For this review, use the dimensioned drawing (mm, ordinates from the lowest corner) and the shaded views. Coordinates: 2 decimals unless noted, no trailing zeros. Loops run counter-clockwise (first coordinate to the right, second up) from the corner with the lowest first, then second, coordinate; pieces in that order, holes last. Notation, with made-up numbers: (10.25, -27) - (50.25, -27) arc R15 ccw to (50.25, -7) - close; hole circle Ø8 at (-7, 46.5). An arc over 180 degrees is marked (long way). One line per item, written item: value. Start each with the question number.
1. We need section C-C, the plane y = 3.9. Give the boundary of the cut face in (x, z).
2. We need section A-A, the plane x = 8.8. Give the boundary of the cut face in (y, z), then the cut area to 3 significant figures.
3. We need section B-B, the plane z = 33.1. Give the boundary of the cut face in (x, y).
4. To check wall thickness, follow line 1 (X direction, y = 0.45, z = 33.1); line 2 (Z direction, x = 8.8, y = 1.35); line 3 (Y direction, x = 1.75, z = 44). State the ranges of each line that lie inside material, in increasing order.
5. Insertion check: P1, Ø1, axis at y = 0.5, z = 12.5, coming from the -X side; P2, Ø10, axis at x = 9, z = 35.5, coming from the +Y side; P3, Ø0.9, axis at y = 3.5, z = 5, coming from the -X side; P4, Ø1.5, axis at y = 3, z = 2, coming from the +X side. Each pin has a flat end and moves straight along its axis. Give the tip position at first contact, or say it passes through.
6. We need section D-D, the plane z = 15. Give the boundary of the cut face in (x, y).
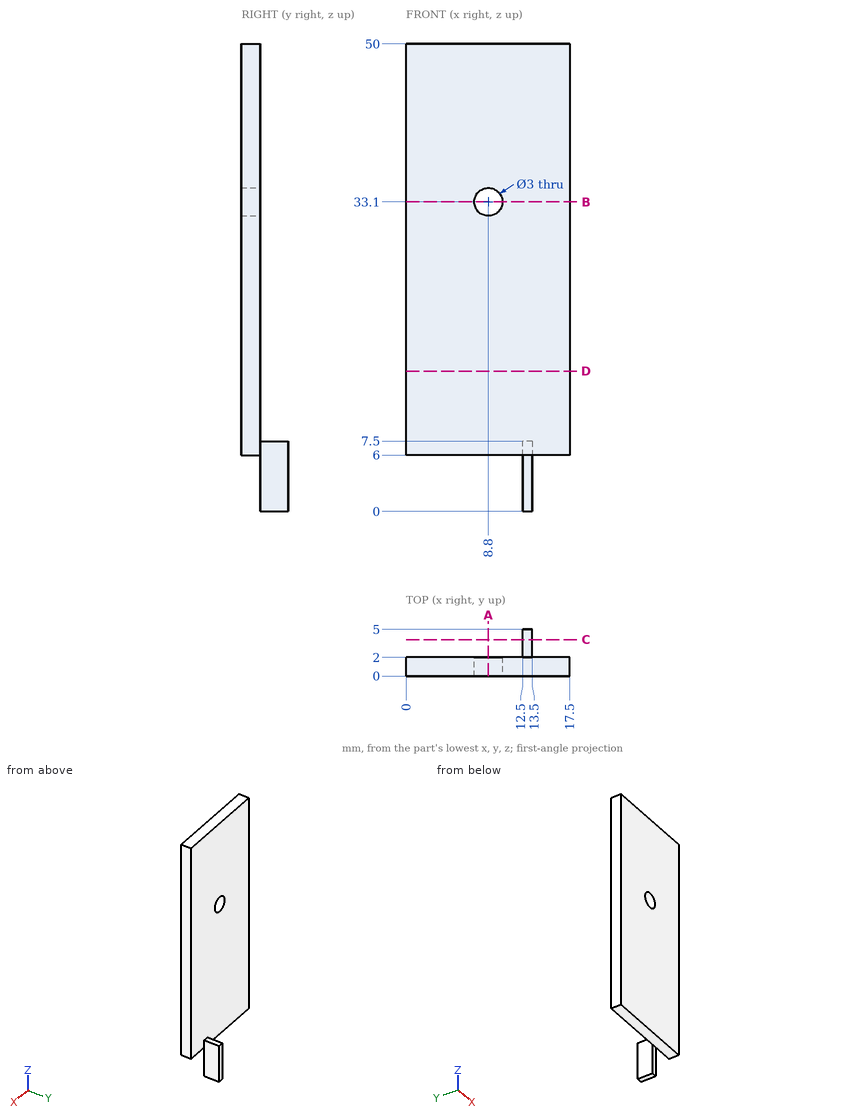
Findings below:
1. outline: (12.5, 0) - (13.5, 0) - (13.5, 7.5) - (12.5, 7.5) - close
2. outline: (0, 6) - (2, 6) - (2, 31.6) - (0, 31.6) - close; (0, 34.6) - (2, 34.6) - (2, 50) - (0, 50) - close
2. area: 82.0 mm2
3. outline: (0, 0) - (7.3, 0) - (7.3, 2) - (0, 2) - close; (10.3, 0) - (17.5, 0) - (17.5, 2) - (10.3, 2) - close
4. line 1: 0 to 7.3, 10.3 to 17.5
4. line 2: 6 to 31.6, 34.6 to 50
4. line 3: 0 to 2
5. P1: x = 0
5. P2: y = 2
5. P3: x = 12.5
5. P4: x = 13.5
6. outline: (0, 0) - (17.5, 0) - (17.5, 2) - (0, 2) - close
